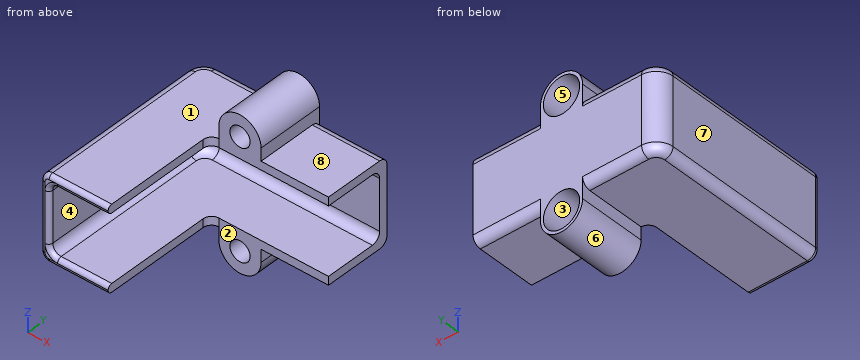
from build123d import *

# Parameters (mm, degrees)
EXTRUDE_1_DEPTH           = 5
EXTRUDE_1_2_DEPTH         = 8
CUT_EXTRUDE_1_DEPTH       = 4
FILLET_1_R                = 2
HOLE_WIZARD_1_D           = 2.4
HOLE_WIZARD_1_DEPTH       = 15
HOLE_WIZARD_1_CBORE_D     = 4.3
HOLE_WIZARD_1_CBORE_DEPTH = 5
HOLE_WIZARD_1_TIP         = 0.721032743
FILLET_2_R                = 1
FILLET_3_R                = 1
FILLET_4_R                = 1
FILLET_5_R                = 0.5
FILLET_6_R                = 0.5


with BuildPart() as part:
    # 草图1 → Extrude 1 (new, symmetric)
    with BuildSketch(Plane.XY):
        Polygon((4, -18), (4, -4), (18, -4), (18, 4), (-4, 4), (-4, -18), align=None)
    extrude(amount=EXTRUDE_1_DEPTH, both=True)

    # 草图3 → Extrude 1 2 (add)
    with BuildSketch(Plane(origin=(0, 4, 0), x_dir=(1, 0, 0), z_dir=(0, 1, 0))):
        with BuildLine():
            Line((10, 6.5), (10, -6.5))
            ThreePointArc((10, -6.5), (7.5, -9), (5, -6.5))
            Line((5, -6.5), (5, 6.5))
            ThreePointArc((5, 6.5), (7.5, 9), (10, 6.5))
        make_face()
    extrude(amount=-EXTRUDE_1_2_DEPTH)

    # 草图2 → 切除-拉伸1 (cut, symmetric)
    with BuildSketch(Plane.XY):
        Polygon((18, 3), (-3, 3), (-3, -18), (4, -18), (4, -4), (18, -4), align=None)
    extrude(amount=CUT_EXTRUDE_1_DEPTH, both=True, mode=Mode.SUBTRACT)

    # 圆角1
    fillet_1_edges = [part.edges().sort_by_distance(p)[0] for p in [
        (-3, 3, 0),
        (-4, 4, 0),
    ]]
    fillet(fillet_1_edges, radius=FILLET_1_R)

    # 打孔尺寸(%根据)内六角圆柱头螺钉的类型1
    with Locations(Plane(origin=(0, 4, 0), x_dir=(1, 0, 0), z_dir=(0, 1, 0))):
        with Locations((7.5, 6.5), (7.5, -6.5)):
            CounterBoreHole(HOLE_WIZARD_1_D / 2, HOLE_WIZARD_1_CBORE_D / 2, HOLE_WIZARD_1_CBORE_DEPTH, depth=HOLE_WIZARD_1_DEPTH)
            with Locations((0, 0, -(HOLE_WIZARD_1_DEPTH + HOLE_WIZARD_1_TIP / 2))):  # 118° drill point
                Cone(0, HOLE_WIZARD_1_D / 2, HOLE_WIZARD_1_TIP, mode=Mode.SUBTRACT)

    # 圆角2
    fillet_2_edges = [part.edges().sort_by_distance(p)[0] for p in [
        (1.5, 4, -5),
        (1.5, 4, 5),
        (8.5, 3, -4),
        (8.5, 3, 4),
        (-4, -8, -5),
        (-4, -8, 5),
        (-3.414213562, 3.414213562, -5),
        (-3.414213562, 3.414213562, 5),
        (-3, -8.5, 4),
        (-3, -8.5, -4),
        (-2.414213562, 2.414213562, 4),
        (-2.414213562, 2.414213562, -4),
    ]]
    fillet(fillet_2_edges, radius=FILLET_2_R)

    # 圆角3
    fillet_3_edges = [part.edges().sort_by_distance(p)[0] for p in [
        (14, 4, 5),
        (14, 4, -5),
    ]]
    fillet(fillet_3_edges, radius=FILLET_3_R)

    # 圆角4
    fillet_4_edges = [part.edges().sort_by_distance(p)[0] for p in [
        (4, -4, -4.5),
        (4, -4, 4.5),
    ]]
    fillet(fillet_4_edges, radius=FILLET_4_R)

    # 圆角5
    fillet_5_edges = [part.edges().sort_by_distance(p)[0] for p in [
        (-4, -18, 0),
        (-3.707106781, -18, -4.707106781),
        (-3.707106781, -18, 4.707106781),
        (0.5, -18, -5),
        (0.5, -18, 5),
    ]]
    fillet(fillet_5_edges, radius=FILLET_5_R)

    # 圆角6
    fillet_6_edges = [part.edges().sort_by_distance(p)[0] for p in [
        (1, -18, -4),
        (-2.707106781, -18, -3.707106781),
        (1, -18, 4),
        (-2.707106781, -18, 3.707106781),
        (-3, -18, 0),
    ]]
    fillet(fillet_6_edges, radius=FILLET_6_R - 0.0001)  # a hair under: the kernel refuses the full size


solid = part.part
Work out the finished part from the listing and answer in its coordinate system (mm). Face numbers are marked on the shaded views. A direction names the side the tool comes from. Coordinates: 2 decimals unless noted, no trailing zeros. Loops run counter-clockwise (first coordinate to the right, second up) from the corner with the lowest first, then second, coordinate; pieces in that order, holes last. Notation, with made-up numbers: (9, 61.5) -> (37, 61.5) arc R21 ccw to (37, 92.5) -> close; hole circle Ø2 at (69.5, 60.5). An arc over 180 degrees is marked (long way). Write each question's results on one line, items separated by ' | '. Start each with the question number.
1) For the marked faces 1, 2, 3 and 4, determine the directions among +Z, -Z, +X, -X, +Y, -Y from which every point of the face is accessible in a straight line to the end or side of a thin tool.
2) The mould has two halves that part along X. Classify the marked faces 5, 6, 7 and 8: pulls with the +X half, pulls with the -X half, needs draft (parallel to the pull), parting line crosses it, or undercut.
3) Find section B-B on x = 12.5. Determine the outline of the cut face in (y, z).
4) Find section A-A on y = -2.25. Determine the outline of the cut face in (x, z), then the cut area to 3 significant figures.
5) Find section C-C on x = 7.5. Determine the outline of the cut face in (y, z).
6) Flat-ended cylindrical pins translate along their axes: P1, Ø0.5, axis at y = -12, z = -4.5, coming from the +X side; P2, Ø1.2, axis at y = 1.5, z = 5, coming from the -X side; P3, Ø10, axis at x = 14, z = -1.5, coming from the -Y side. Find the tip coordinate at first contact, or state that the pin passes through.
7) Consider line 1 along Z through (x, y) = (7.5, 0.15); line 2 along Z through (x, y) = (2.5, 0.5); line 3 along X through (y, z) = (-2.9, -6.5). Determine where each line is inside the solid, lowest interval first.
Response values:
1) face 1: +Z, -X, +Y, -Y | face 2: +Z, -Z, +X, -Y | face 3: +Y | face 4: +X, -Y
2) face 5: undercut | face 6: parting line crosses it | face 7: pulls with the -X half | face 8: needs draft
3) outline: (-4, -5) -> (3, -5) arc R1 ccw to (4, -4) -> (4, 4) arc R1 ccw to (3, 5) -> (-4, 5) -> (-4, 4) -> (2, 4) arc R1 cw to (3, 3) -> (3, -3) arc R1 cw to (2, -4) -> (-4, -4) -> close
4) outline: (-4, -4) arc R1 ccw to (-3, -5) -> (5, -5) -> (5, -6.5) arc R2.5 ccw to (10, -6.5) -> (10, -5) -> (18, -5) -> (18, -4) -> (-2, -4) arc R1 cw to (-3, -3) -> (-3, 3) arc R1 cw to (-2, 4) -> (18, 4) -> (18, 5) -> (10, 5) -> (10, 6.5) arc R2.5 ccw to (5, 6.5) -> (5, 5) -> (-3, 5) arc R1 ccw to (-4, 4) -> close; hole circle Ø2.4 at (7.5, -6.5); hole circle Ø2.4 at (7.5, 6.5) | area: 77.6 mm^2
5) outline: (-4, -9) -> (4, -9) -> (4, -8.65) -> (-1, -8.65) -> (-1, -7.7) -> (-4, -7.7) -> close; (-4, -5.3) -> (-1, -5.3) -> (-1, -4.35) -> (4, -4.35) -> (4, 4.35) -> (-1, 4.35) -> (-1, 5.3) -> (-4, 5.3) -> (-4, 4) -> (2, 4) arc R1 cw to (3, 3) -> (3, -3) arc R1 cw to (2, -4) -> (-4, -4) -> close; (-4, 7.7) -> (-1, 7.7) -> (-1, 8.65) -> (4, 8.65) -> (4, 9) -> (-4, 9) -> close
6) P1: stops at x = 4 | P2: stops at x = -3.92 | P3: stops at y = -4
7) line 1: z = -9 to -8.65, -4.35 to -4, 4 to 4.35, 8.65 to 9 | line 2: z = -5 to -4, 4 to 5 | line 3: x = 5 to 6.3, 8.7 to 10
